```python
from build123d import *

# Parameters (mm, degrees)
SKETCH1_W                = 40
SKETCH1_H                = 40
BOSS_EXTRUDE1_DEPTH      = 7.5
SKETCH2_R                = 8.5
CUT_EXTRUDE1_DEPTH       = 20
CUT_EXTRUDE1_DEPTH_BACK  = 20
F_8_0_8_DIAMETER_HOLE1_D = 8


with BuildPart() as part:
    # Sketch1 → Boss-Extrude1 (new body)
    with BuildSketch(Plane(origin=(0, 0, 0), x_dir=(1, 0, 0), z_dir=(0, 1, 0))):
        Rectangle(SKETCH1_W, SKETCH1_H)
    extrude(amount=BOSS_EXTRUDE1_DEPTH)

    # Sketch2 → Cut-Extrude1 (cut, two sides)
    with BuildSketch(Plane(origin=(0, 0, 0), x_dir=(0, 0, -1), z_dir=(1, 0, 0))) as cut_extrude1_sk:
        with Locations((0, 10)):
            Circle(SKETCH2_R)
    extrude(amount=CUT_EXTRUDE1_DEPTH, mode=Mode.SUBTRACT)
    extrude(cut_extrude1_sk.sketch, amount=-CUT_EXTRUDE1_DEPTH_BACK, mode=Mode.SUBTRACT)

    # 8.0 _8_ Diameter Hole1 (through all)
    with Locations(Plane(origin=(0, 7.5, 0), x_dir=(1, 0, 0), z_dir=(0, 1, 0))):
        with Locations((1.247226864, 14.667228454), (0, -14.232771546)):
            Hole(F_8_0_8_DIAMETER_HOLE1_D / 2)


solid = part.part
```
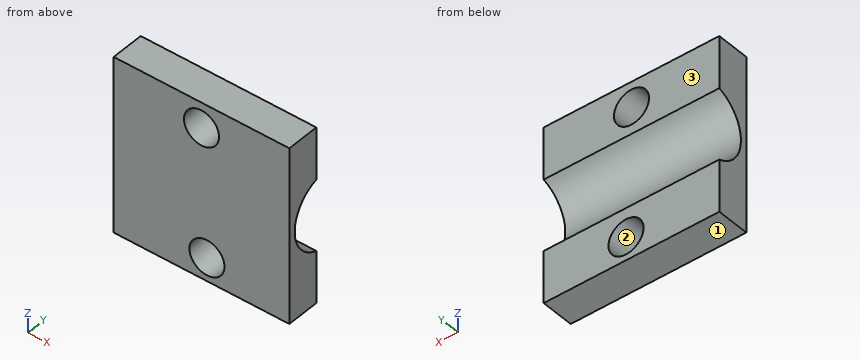
Could you check a few things on this model? Use its own coordinates, in mm. Face numbers are marked on the shaded views. Round coordinates to 2 decimals unless told otherwise and drop trailing zeros. Write each loop counter-clockwise with the first axis right and the second up, starting at its lowest first coordinate (ties: lowest second). Pieces come first, ordered by that corner, then holes. Notation, with made-up numbers: M -1,50 L 8,50 A13 ccw 8,60 Z; hole C 34.25,78.25 d4. An arc over 180 degrees is marked long. Answer in a Markdown table with one row per item. Add a question column.
Q1. Will this pin go through, and if not, where does the flat tip stop? pin 1 Ø1 at (x, z) = (-9, -2) entering from +Y.
Q2. Imagine slicing it at C-C (z = -16). Please give me the cut outline in (x, y).
Q3. Imagine slicing it at D-D (x = -13). Please give me the cut outline in (y, z), then the cut area to 3 significant figures.
Q4. Imagine slicing it at A-A (y = 4.75). Please give me the cut outline in (x, z).
Q5. If I drill on line 1 (Z direction, x = 1, y = 3); line 2 (Z direction, x = 0, y = 2.25); line 3 (X direction, y = 6.5, z = 14), over which ranges is the centre line in solid material (lowest first)? Write a range as from..to.
Q6. Imagine slicing it at B-B (x = 3). Please give me the cut outline in (y, z).
Q7. If we mould it in two halves opening along Z, with no side actions, what happens to the marked faces 1, 2 and 3? For each: +Z half, -Z half, draft (parallel to the pull), parting line (faces both ways), or undercut.
Values:
| question | item | result |
|---|---|---|
| 1 | pin 1 | y = 1.88 |
| 2 | outline | M -20,0 L -2.52,0 L -2.52,7.5 L -20,7.5 Z; M 5.02,0 L 20,0 L 20,7.5 L 5.02,7.5 Z |
| 3 | outline | M 0,-20 L 7.5,-20 L 7.5,-8.12 A8.5 cw 7.5,8.12 L 7.5,20 L 0,20 Z |
| 3 | area | 228 mm^2 |
| 4 | outline | M -20,-20 L 20,-20 L 20,-6.68 L -20,-6.68 Z; M -20,6.68 L 20,6.68 L 20,20 L -20,20 Z; hole C 0,14.23 d8; hole C 1.25,-14.67 d8 |
| 5 | line 1 | -20..-18.66, -10.67..-4.82, 4.82..10.36, 18.11..20 |
| 5 | line 2 | -20..-18.47, -10.87..-3.49, 3.49..10.23, 18.23..20 |
| 5 | line 3 | -20..-3.99, 3.99..20 |
| 6 | outline | M 0,-20 L 7.5,-20 L 7.5,-18.26 L 0,-18.26 Z; M 0,-11.07 L 7.5,-11.07 L 7.5,-8.12 A8.5 cw 7.5,8.12 L 7.5,11.59 L 0,11.59 Z; M 0,16.88 L 7.5,16.88 L 7.5,20 L 0,20 Z |
| 7 | face 1 | -Z half |
| 7 | face 2 | undercut |
| 7 | face 3 | draft |
